Input: part model. Units: mm. Frame: model coordinates. Round coordinates to 2 decimals unless told otherwise and drop trailing zeros. Loops run counter-clockwise (first coordinate to the right, second up) from the corner with the lowest first, then second, coordinate; pieces in that order, holes last. Notation, with made-up numbers: M 57.25,-1 L 111.25,-1 A19 cw 111.25,25 Z; hole C 49,88.5 d11. An arc over 180 degrees is marked long. Put each result on its own line as item: value. Start each with the question number.
1) Draft query along Z for faces 1 (the face through (126, -6, 278)), 2 (the face through (64.82, -52.26, -291.89)), 3 (the face through (304.705, -56.7, -13.41)). Return one class per face: +Z half, -Z half, draft (parallel to the pull), parting line (faces both ways), or undercut.
2) Line query: probe 1 along Y at (x, z) = (-323, -221.5); probe 2 along Z at (x, y) = (-168.5, -98); probe 3 along Z at (x, y) = (-4.5, -8). Output: solid intervals per line, ascending.
3) Pin query (flat end, axial travel): pin 1 (8.5 mm diameter, centred on x = 236.88, z = 236.88, fed in from -Y); pin 2 (23 mm diameter, centred on x = -100.94, z = 376.71, fed in from +Y); pin 3 (12 mm diameter, centred on x = 132.5, y = -72.5, fed in from -Z); pin 4 (2 mm diameter, centred on x = 47.5, y = -49.5, fed in from +Z). Return the tip coordinate at first contact, or that it passes through.
4) Section B-B on y = -76.5. Output: boundary loops of the cut face in (x, z), plus the area to 3 significant figures.
5) Section A-A on z = 140.5. Output: boundary loops of the cut face in (x, y), plus the area to 3 significant figures.
Autodesk Inventor part; units mm, degrees
ref_plane "YZ Plane" through (0, 0, 0) normal (1, 0, 0) x (0, 1, 0)
ref_plane "XZ Plane" through (0, 0, 0) normal (0, 1, 0) x (-1, 0, 0)
ref_plane "XY Plane" through (0, 0, 0) normal (0, 0, 1) x (1, 0, 0)
sketch "Sketch1" plane through (0, 0, 0) normal (0, 0, 1) x (1, 0, 0)
  line L0 (-299, -106) -> (-299, 0)
  line L1 (-299, 0) -> (-420, 0)
  line L2 (-420, 0) -> (-420, -6)
  line L3 (-420, -6) -> (-305, -6)
  line L4 (-305, -6) -> (-305, -106)
  line L5 (-305, -106) -> (-299, -106)
  line L6 (0, 0) -> (0, -106)
  dimension "d0" = 6
  dimension "d1" = 6
  dimension "d2" = 610
  dimension "d3" = 840
  dimension "d4" = 100
revolve "Revolution1" add sketch "Sketch1" angle 360 about axis through (0, 0, 0) along (0, -1, 0)
sketch "Sketch2" plane through (0, 0, 0) normal (0, 1, 0) x (1, 0, 0)
  circle A0 centre (-335, 0) radius 7.1437
  circle A1 centre (-390, 0) radius 7.1437
  circle A2 centre (0, 0) radius 335 construction
  circle A3 centre (0, 0) radius 390 construction
  dimension "d9" = 670
  dimension "d10" = 780
  dimension "d6" = 14.2875
  dimension "d7" = 14.2875
extrude "Extrusion1" cut sketch "Sketch2" against normal through all
pattern_circular "Circular Pattern1" count 24 over 360 about axis through (0, -53, 0) along (0, 1, 0) of "Extrusion1"
equation "\"d1\" = d0"
equation "\"d7\" = d6"
properties part number "Brida_cuello_tapa" material "Steel ASTM A36"
Geometry results:
1. face 1: draft
1. face 2: undercut
1. face 3: parting line
2. probe 1: y = -6 to 0
2. probe 2: z = -254.23 to -247, 247 to 254.23
2. probe 3: z = -304.97 to -298.97, 298.97 to 304.97
3. pin 1: passes through
3. pin 2: stops at y = 0
3. pin 3: stops at z = -277.53
3. pin 4: stops at z = 301.43
4. outline: C 0,0 d610; hole C 0,0 d598
4. area: 11,400 mm²
5. outline: M -395.8,-6 L -270.71,-6 L -270.71,-106 L -263.93,-106 L -263.93,0 L -395.8,0 Z; M 263.93,-106 L 270.71,-106 L 270.71,-6 L 395.8,-6 L 395.8,0 L 263.93,0 Z
5. area: 2,940 mm²
